from build123d import *

# Parameters (mm, degrees)
BOSS_EXTRUDE1_DEPTH = 2.3622


with BuildPart() as part:
    # Sketch1 → Boss-Extrude1 (new body)
    with BuildSketch(Plane(origin=(0, 0, 0), x_dir=(1, 0, 0), z_dir=(0, 1, 0))):
        with BuildLine():
            Line((2.055202021, 14.546975478), (2.055202021, 5.72400467))
            Line((2.055202021, 5.72400467), (-13.894021226, 4.719731013))
            ThreePointArc((-13.894021226, 4.719731013), (-14.998563485, 3.466742259), (-13.745574731, 2.3622))
            Line((-13.745574731, 2.3622), (2.129425269, 3.361800046))
            ThreePointArc((2.129425269, 3.361800046), (3.201004497, 2.477166942), (2.3876, 1.350565462))
            Line((2.3876, 1.350565462), (2.3876, 1.846546672))
            Line((2.3876, 1.846546672), (0, 1.846546672))
            Line((0, 1.846546672), (0, 0))
            Line((0, 0), (-0.956548556, 0))
            Line((-0.956548556, 0), (-1.436625807, 0.480077251))
            Line((-1.436625807, 0.480077251), (-1.916703058, 0))
            Line((-1.916703058, 0), (-74.6432929, 0))
            Line((-74.6432929, 0), (-75.123370151, 0.480077251))
            Line((-75.123370151, 0.480077251), (-75.603447402, 0))
            Line((-75.603447402, 0), (-76.559995958, 0))
            Line((-76.559995958, 0), (-76.559995958, 1.846546672))
            Line((-76.559995958, 1.846546672), (-78.947595958, 1.846546672))
            Line((-78.947595958, 1.846546672), (-78.947595958, 1.350565462))
            ThreePointArc((-78.947595958, 1.350565462), (-79.761000455, 2.477166942), (-78.689421226, 3.361800046))
            Line((-78.689421226, 3.361800046), (-62.814421226, 2.3622))
            ThreePointArc((-62.814421226, 2.3622), (-61.561432472, 3.466742259), (-62.665974731, 4.719731013))
            Line((-62.665974731, 4.719731013), (-78.615197979, 5.72400467))
            Line((-78.615197979, 5.72400467), (-78.615197979, 14.546975478))
            Line((-78.615197979, 14.546975478), (-75.998997979, 14.546975478))
            Line((-75.998997979, 14.546975478), (-75.998997979, 21.582775478))
            Line((-75.998997979, 21.582775478), (-69.648997979, 21.582775478))
            Line((-69.648997979, 21.582775478), (-69.648997979, 14.546975478))
            Line((-69.648997979, 14.546975478), (-53.215197979, 14.546975478))
            Line((-53.215197979, 14.546975478), (-53.215197979, 21.806295525))
            Line((-53.215197979, 21.806295525), (-46.865197979, 21.806295525))
            Line((-46.865197979, 21.806295525), (-46.865197979, 12.967095525))
            Line((-46.865197979, 12.967095525), (-29.694797979, 12.967095525))
            Line((-29.694797979, 12.967095525), (-29.694797979, 21.806295525))
            Line((-29.694797979, 21.806295525), (-23.344797979, 21.806295525))
            Line((-23.344797979, 21.806295525), (-23.344797979, 14.546975478))
            Line((-23.344797979, 14.546975478), (-6.910997979, 14.546975478))
            Line((-6.910997979, 14.546975478), (-6.910997979, 21.582775478))
            Line((-6.910997979, 21.582775478), (-0.560997979, 21.582775478))
            Line((-0.560997979, 21.582775478), (-0.560997979, 14.546975478))
            Line((-0.560997979, 14.546975478), (2.055202021, 14.546975478))
        make_face()
    extrude(amount=BOSS_EXTRUDE1_DEPTH)


solid = part.part
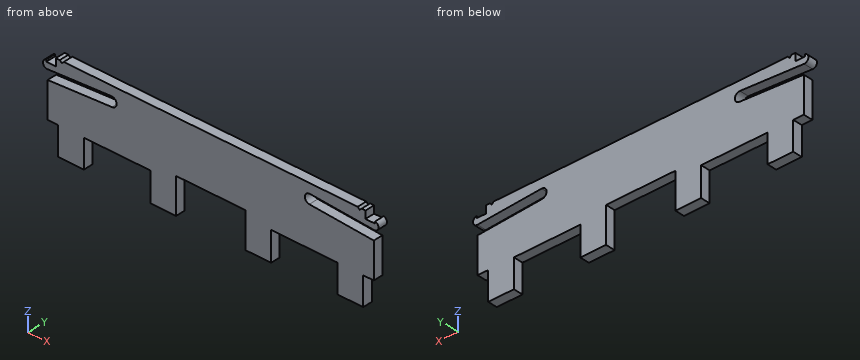
Read the model definition and answer for the solid it produces. Units are mm, in the model's axes. Round coordinates to 2 decimals unless told otherwise and drop trailing zeros. Write each loop counter-clockwise with the first axis right and the second up, starting at its lowest first coordinate (ties: lowest second). Pieces come first, ordered by that corner, then holes.
1. The part is cut by section A-A, the plane z = -19.5. Determine the outline of the cut face in (x, y), then the cut area to 3 significant figures.
2. The part is cut by section B-B, the plane x = -13. Determine the outline of the cut face in (y, z).
3. Straight lines are drawn through the part: L1, parallel to X at y = 2.2, z = -18.25; L2, parallel to X at y = 1, z = -1.5; L3, parallel to X at y = 0.6, z = -8. For each, find the intervals that lie inside material, in ascending order.
4. The part is cut by section C-C, the plane z = -10.75. Determine the outline of the cut face in (x, y).
5. Given pin 1 Ø0.7 at (y, z) = (1, -16.5) entering from -X; pin 2 Ø0.7 at (x, y) = (1, 1) entering from -Z; pin 3 Ø1 at (x, y) = (-7, 1.5) entering from -Z, each flat-ended and moving along its own axis, determine where each tip first touches the part or whether it passes through.
6. The part is cut by section D-D, the plane x = -55. Determine the outline of the cut face in (y, z), then the cut area to 3 significant figures.
Values:
1. outline: (-76, 0) - (-69.65, 0) - (-69.65, 2.36) - (-76, 2.36) - close; (-53.22, 0) - (-46.87, 0) - (-46.87, 2.36) - (-53.22, 2.36) - close; (-29.69, 0) - (-23.34, 0) - (-23.34, 2.36) - (-29.69, 2.36) - close; (-6.91, 0) - (-0.56, 0) - (-0.56, 2.36) - (-6.91, 2.36) - close
1. area: 60.0 mm2
2. outline: (0, -14.55) - (2.36, -14.55) - (2.36, -4.78) - (0, -4.78) - close; (0, -2.41) - (2.36, -2.41) - (2.36, 0) - (0, 0) - close
3. L1: x = -76 to -69.65, -53.22 to -46.87, -29.69 to -23.34, -6.91 to -0.56
3. L2: x = -79.31 to -78.95, -76.56 to 0, 2.39 to 2.75
3. L3: x = -78.62 to 2.06
4. outline: (-78.62, 0) - (2.06, 0) - (2.06, 2.36) - (-78.62, 2.36) - close
5. pin 1: stops at x = -76
5. pin 2: stops at z = -14.55
5. pin 3: stops at z = -21.58
6. outline: (0, -14.55) - (2.36, -14.55) - (2.36, 0) - (0, 0) - close
6. area: 34.4 mm2
